from build123d import *

# Parameters (mm, degrees)
F0_R     = 4.5
F1_DEPTH = 20
F2_SIZE2 = 1.5
F2_SIZE  = 5
F3_D     = 5


with BuildPart() as f1:
    # F0 (on Top) → F1 (new body)
    with BuildSketch(Plane.XY):
        Circle(F0_R)
    extrude(amount=F1_DEPTH)

    # F2
    f2_edges = [f1.edges().sort_by_distance(p)[0] for p in [
        (-4.5, 0, 20),
    ]]
    f2_side = f1.faces().sort_by_distance((-4.5, 0, 10))[0]
    chamfer(f2_edges, length=F2_SIZE, length2=F2_SIZE2, reference=f2_side)

    # F3 (through all)
    with Locations(Plane(origin=(0, 0, 0), x_dir=(1, 0, 0), z_dir=(0, 0, -1))):
        with Locations((0, 0)):
            Hole(F3_D / 2)


solid = f1.part
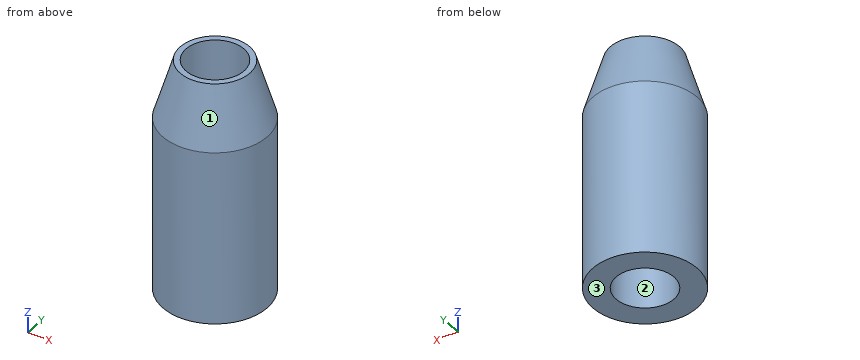
Design review of the part built by this model. Coordinates are the model's own, in mm. Face numbers are marked on the shaded views. Give positions to 0.01 mm unless a question says otherwise; leave off trailing zeros. Loops run counter-clockwise (first coordinate to the right, second up) from the corner with the lowest first, then second, coordinate; pieces in that order, holes last. Notation, with made-up numbers: (25, 39.5) - (83, 39.5) arc R14 cw to (83, 64.5) - close; hole circle Ø2 at (-25, 24.25). An arc over 180 degrees is marked (long way). Write item = value, one per line.
1) Clearance check with flat-ended pins moving along their axes: pin 1 Ø5 at (x, y) = (2, -3.5) entering from +Z; pin 2 Ø2 at (x, z) = (-2.5, 7) entering from +Y; pin 3 Ø1.5 at (x, z) = (3, 15.5) entering from -Y. State where each tip first meets the part, or that it passes through.
Result sheet:
pin_1 = 20
pin_2 = 4.24
pin_3 = -3.79
2) Take a section at A-A on y = 0. State the section outline as (x, z) points, and give its area (3 significant figures).
Result sheet:
outline = (-4.5, 0) - (-2.5, 0) - (-2.5, 20) - (-3, 20) - (-4.5, 15) - close; (2.5, 0) - (4.5, 0) - (4.5, 15) - (3, 20) - (2.5, 20) - close
area = 72.5 mm2
3) Take a section at D-D on z = 5.5. State the section outline as (x, y) points.
Result sheet:
outline = circle Ø9 at (0, 0); hole circle Ø5 at (0, 0)
4) Draft analysis for pull direction X (two halves, no side actions). For the marked faces 1, 2 and 3, state which applies: +X half, -X half, draft (parallel to the pull), parting line (faces both ways), or undercut.
Result sheet:
face_1 = parting line
face_2 = undercut
face_3 = draft
5) To check wall thickness, follow line 1 (Y direction, x = 0, z = 9.5); line 2 (X direction, y = 2.25, z = 6.5); line 3 (Y direction, x = 1.75, z = 1.5). State the ranges of each line that lie inside material, in increasing order.
Result sheet:
line_1 = -4.5 to -2.5, 2.5 to 4.5
line_2 = -3.9 to -1.09, 1.09 to 3.9
line_3 = -4.15 to -1.79, 1.79 to 4.15
6) Take a section at C-C on z = 15.5. State the section outline as (x, y) points.
Result sheet:
outline = circle Ø8.7 at (0, 0); hole circle Ø5 at (0, 0)
